Autodesk Inventor part; units mm, degrees
ref_plane "YZ Plane" through (0, 0, 0) normal (1, 0, 0) x (0, 1, 0)
ref_plane "XZ Plane" through (0, 0, 0) normal (0, 1, 0) x (-1, 0, 0)
ref_plane "XY Plane" through (0, 0, 0) normal (0, 0, 1) x (1, 0, 0)
sketch "Sketch1" plane through (0, 0, 0) normal (1, 0, 0) x (0, 1, 0)
  line L0 (-32, 106) -> (32, 106)
  line L1 (32, 106) -> (32, -106)
  line L2 (32, -106) -> (-32, -106)
  line L3 (-32, -106) -> (-32, 106)
  line L4 (-32, 106) -> (32, -106) construction
  line L5 (32, 106) -> (-32, -106) construction
  point P0 (0, 0)
  dimension "d0" = 64
  dimension "d1" = 212
extrude "Extrusion1" add sketch "Sketch1" along normal blind 3.175
chamfer "Chamfer1" distance 4 angle 45 2 edges at (1.5875, 32, 106) (1.5875, 32, -106)
chamfer "Chamfer2" distance 4 angle 45 2 edges at (1.5875, -32, 106) (1.5875, -32, -106)
sketch "Sketch3" plane through (3.175, 0, 0) normal (1, 0, 0) x (0, 0, -1)
  circle A0 centre (-84, -8) radius 7 construction
  circle A1 centre (-68, -24) radius 2
  line L0 (-102, -32) -> (102, -32) construction
  line L1 (-84, -1) -> (-84, -15) construction
  circle A2 centre (-100, -24) radius 2
  line L2 (102, 32) -> (-102, 32) construction
  line L3 (0, 32) -> (0, -32) construction
  circle A3 centre (68, -24) radius 2
  circle A4 centre (100, -24) radius 2
  point P0 (0, 0)
  dimension "d22" = 14
  dimension "d23" = 84
  dimension "d24" = 4
  dimension "d25" = 16
  dimension "d26" = 8
  dimension "d27" = 16
extrude "Extrusion3" cut sketch "Sketch3" against normal through all
sketch "Sketch4" plane through (3.175, 0, 0) normal (1, 0, 0) x (0, 0, -1)
  circle A0 centre (-72, 0) radius 7
  point P0 (0, 0)
  dimension "d30" = 14
  dimension "d31" = 72
extrude "Extrusion4" cut sketch "Sketch4" against normal through all
sketch "Sketch6" plane through (3.175, 0, 0) normal (1, 0, 0) x (0, 0, -1)
  circle A0 centre (-72, 0) radius 7 construction
  circle A1 centre (84, 0) radius 7
  line L0 (84, 0) -> (91, 0) construction
  circle A2 centre (76, 8) radius 2
  circle A3 centre (76, -8) radius 2
  circle A4 centre (92, -8) radius 2
  circle A5 centre (92, 8) radius 2
  circle A6 centre (36, 0) radius 7
  circle A7 centre (28, 8) radius 2
  circle A8 centre (28, -8) radius 2
  circle A9 centre (44, -8) radius 2
  circle A10 centre (44, 8) radius 2
  point P0 (0, 0)
  dimension "d65" = 14
  dimension "d67" = 84
  dimension "d71" = 4
  dimension "d72" = 8
  dimension "d73" = 8
  dimension "d76" = 360
  dimension "d78" = 14
  dimension "d79" = 36
  dimension "d80" = 4
  dimension "d81" = 8
  dimension "d82" = 8
  dimension "d85" = 360
extrude "Extrusion6" cut sketch "Sketch6" against normal blind 10
sketch "Sketch8" plane through (3.175, 0, 0) normal (1, 0, 0) x (0, 0, -1)
  circle A0 centre (-98, 28) radius 2
  line L0 (102, 32) -> (-102, 32) construction
  line L1 (-106, 28) -> (-106, -28) construction
  circle A1 centre (-82, 28) radius 2
  circle A2 centre (-66, 28) radius 2
  circle A3 centre (-50, 28) radius 2
  circle A4 centre (-34, 28) radius 2
  circle A5 centre (-18, 28) radius 2
  line L2 (0, 32) -> (0, -32) construction
  line L3 (-102, -32) -> (102, -32) construction
  circle A6 centre (98, 28) radius 2
  circle A7 centre (82, 28) radius 2
  circle A8 centre (66, 28) radius 2
  circle A9 centre (50, 28) radius 2
  circle A10 centre (34, 28) radius 2
  circle A11 centre (18, 28) radius 2
  point P0 (0, 0)
  dimension "d87" = 4
  dimension "d88" = 4
  dimension "d89" = 8
  dimension "d92" = 16
extrude "Extrusion7" cut sketch "Sketch8" against normal through all
sketch "Sketch9" plane through (3.175, 0, 0) normal (1, 0, 0) x (0, 0, -1)
  line L0 (-102, -32) -> (102, -32) construction
  line L1 (-64, -32) -> (-64, -32)
  line L2 (-54, -22) -> (54, -22)
  line L3 (64, -32) -> (64, -32)
  line L4 (-64, -32) -> (64, -32)
  line L5 (-54, -22) -> (-64, -32)
  line L6 (54, -22) -> (64, -32)
  point P0 (0, 0)
  point P1 (-64, -22)
  point P2 (64, -22)
  dimension "d99" = 64
  dimension "d100" = 64
  dimension "d101" = 10
  dimension "d102" = 10
  dimension "d103" = 10
  dimension "d104" = 10
  dimension "d105" = 10
extrude "Extrusion8" cut sketch "Sketch9" against normal through all
sketch "Sketch10" plane through (3.175, 0, 0) normal (1, 0, 0) x (0, 0, -1)
  line L0 (-54, -22) -> (54, -22) construction
  line L1 (-28, -22) -> (-28, -22)
  line L2 (-20, -14) -> (20, -14)
  line L3 (28, -22) -> (28, -22)
  line L4 (-28, -22) -> (28, -22)
  line L5 (-20, -14) -> (-28, -22)
  line L6 (20, -14) -> (28, -22)
  point P0 (0, 0)
  point P1 (-28, -14)
  point P2 (28, -14)
  point P3 (0, -14)
  point P4 (0, -22)
  point P5 (28, -22)
  dimension "d108" = 8
  dimension "d109" = 56
  dimension "d110" = 8
  dimension "d111" = 8
  dimension "d112" = 8
  dimension "d113" = 8
extrude "Extrusion9" cut sketch "Sketch10" against normal through all
properties part number "ArmSidePlate_Template"
Geometry check sheet. Reference: the model listing, model coordinates, mm. A direction names the side the tool comes from. Give positions to 0.01 mm unless a question says otherwise; leave off trailing zeros. Order: outer loops, then holes, each group sorted by start corner. A loop starts at its lowest first (then second) coordinate and runs counter-clockwise, first axis right, second up. Notation, with made-up numbers: (58.5, -11) - (73.5, -11) arc R23 ccw to (73.5, 27) - close; hole circle Ø10 at (78, 85). An arc over 180 degrees is marked (long way). Answer in a Markdown table with one row per item. Add a question column.
Q1. Material ranges on probe 1 along Y at (x, z) = (2.4, -44); probe 2 along Y at (x, z) = (1.85, 50); probe 3 along Y at (x, z) = (0.95, 72), recorded low to high. Write a range as from..to.
Q2. Cross-section at A-A, the plane z = 18. Enter the section's corners in (x, y) (3 decimals).
Q3. Cross-section at D-D, the plane z = 50. Enter the section's corners in (x, y) (3 decimals), then the cut area to 3 significant figures.
Q4. Mould release check, pull along Z, two halves, no side actions. Record for faces 3 (the flat face through (2, 30, 104)), 4 (the cylindrical face through (1.61, -23.399, -101.908)), 5 (the flat face through (3.175, 0, 1)): pulls with the +Z half, pulls with the -Z half, needs draft (parallel to the pull), parting line crosses it, or undercut.
Q5. Gauge pin test, flat ends, axial feed: pin 1 (3.5 mm diameter, centred on y = 28, z = -34, fed in from -X); pin 2 (6.5 mm diameter, centred on y = 8, z = -92, fed in from -X); pin 3 (1 mm diameter, centred on x = 2, z = 1, fed in from -Y). Record the tip position at first contact, or that the pin passes through.
Q6. Cross-section at B-B, the plane x = 2.65. Count the separate pieces of the cut face and the enclosed holes in it, then the cut area to 3 significant figures.
Q7. Tool access check on faces 1 (the cylindrical face through (1.61, -7.399, -77.908)), 2 (the flat face through (2, -18, 24)). Record the directions out of +Z, -Z, +X, -X, +Y, -Y that give a thin tool (end or side, any length) a straight path to the whole face; none if there is none.
Q8. Cross-section at C-C, the plane y = -3. Enter the section's corners in (x, z) (3 decimals).
Check values:
| question | item | result |
|---|---|---|
| 1 | probe 1 | y = -22..-10, -6..6, 10..32 |
| 1 | probe 2 | y = -22..26, 30..32 |
| 1 | probe 3 | y = -32..-7, 7..32 |
| 2 | outline | (0, -14) - (3.175, -14) - (3.175, 26) - (0, 26) - close; (0, 30) - (3.175, 30) - (3.175, 32) - (0, 32) - close |
| 3 | outline | (0, -22) - (3.175, -22) - (3.175, 26) - (0, 26) - close; (0, 30) - (3.175, 30) - (3.175, 32) - (0, 32) - close |
| 3 | area | 159 mm^2 |
| 4 | face 3 | pulls with the +Z half |
| 4 | face 4 | undercut |
| 4 | face 5 | needs draft |
| 5 | pin 1 | passes through |
| 5 | pin 2 | stops at x = 0 |
| 5 | pin 3 | stops at y = -14 |
| 6 | separate pieces | 1 |
| 6 | enclosed holes | 27 |
| 6 | area | 11,200 mm^2 |
| 7 | face 1 | +X, -X |
| 7 | face 2 | +X, -X, -Y |
| 8 | outline | (0, -106) - (3.175, -106) - (3.175, -90.325) - (0, -90.325) - close; (0, -77.675) - (3.175, -77.675) - (3.175, -42.325) - (0, -42.325) - close; (0, -29.675) - (3.175, -29.675) - (3.175, 65.675) - (0, 65.675) - close; (0, 78.325) - (3.175, 78.325) - (3.175, 106) - (0, 106) - close |
